from build123d import *

# Parameters (mm, degrees)
SALIENTE_EXTRUIR1_DEPTH = 5
CROQUIS2_R              = 2.5
SALIENTE_EXTRUIR2_DEPTH = 5
CROQUIS3_R              = 5
SALIENTE_EXTRUIR3_DEPTH = 10


with BuildPart() as part:
    # Croquis1 → Saliente-Extruir1 (new body)
    with BuildSketch(Plane.XY):
        with BuildLine():
            Line((-52.49750025, 5), (52.49750025, 5))
            Line((52.49750025, 5), (72.49750025, -10))
            Line((72.49750025, -10), (72.49750025, -25.5))
            Line((72.49750025, -25.5), (62.49750025, -25.5))
            Line((62.49750025, -25.5), (62.49750025, -12.5))
            Line((62.49750025, -12.5), (52.49750025, -5))
            Line((52.49750025, -5), (-52.49750025, -5))
            ThreePointArc((-52.49750025, -5), (-103.00249975, 0), (-52.49750025, 5))
        make_face()
    extrude(amount=SALIENTE_EXTRUIR1_DEPTH)

    # Croquis2 → Saliente-Extruir2 (add)
    with BuildSketch(Plane.XY.offset(5)):
        with Locations((-77.50249975, 12.5)):
            Circle(CROQUIS2_R)
    extrude(amount=SALIENTE_EXTRUIR2_DEPTH)

    # Croquis3 → Saliente-Extruir3 (add)
    with BuildSketch(Plane.XY.offset(5)):
        with Locations((-77.50249975, 0)):
            Circle(CROQUIS3_R)
    extrude(amount=SALIENTE_EXTRUIR3_DEPTH)


solid = part.part
Geometry check sheet. Reference: the model listing, model coordinates, mm. A direction names the side the tool comes from. Round coordinates to 2 decimals unless told otherwise and drop trailing zeros. Write each loop counter-clockwise with the first axis right and the second up, starting at its lowest first coordinate (ties: lowest second). Pieces come first, ordered by that corner, then holes. Notation, with made-up numbers: (-35, 76.5) -> (-28, 76.5) arc R25 cw to (-28, 93.5) -> close; hole circle Ø3 at (-20.5, -17.5). An arc over 180 degrees is marked (long way). One line per item, written item: value. Start each with the question number.
(1) Cross-section at D-D, the plane y = 18.5. Record the cut outline in (x, z).
(2) Access from +Z, -Z, +X, -X, +Y, -Y to the whole of each face (thin tool, end or side, straight path). Record for faces 4 (the flat face through (-78, 13, 10)), 5 (the cylindrical face through (-82.5, 0.2, 9.9)), 6 (the flat face through (57.568, -8.802, 2.465)).
(3) Cross-section at A-A, the plane z = 2.5. Record the cut outline in (x, y), and give its area (3 significant figures).
(4) Cross-section at C-C, the plane x = -40. Record the cut outline in (y, z), and give its area (3 significant figures).
(5) Scan lines: line 1 (Z direction, x = 14.5, y = -4.5); line 2 (Y direction, x = -22, z = 1.5); line 3 (X direction, y = -13.5, z = 2.5). Record each from-to range of solid material in increasing order. Write a range as [from, to].
(6) Draft check along Y on faces 1 (the cylindrical face through (-79.5, 11, 7.5)), 2 (the flat face through (-1, 5, 2)), 3 (the flat face through (62.498, -19, 2)). Enter one of: +Y half, -Y half, draft (parallel to the pull), parting line (faces both ways), or undercut.
(7) Cross-section at B-B, the plane y = 3. Record the cut outline in (x, z).
(8) Go/stop test with flat-tipped pins: pin 1 Ø2.5 at (x, z) = (-21.5, 3.5) entering from -Y; pin 2 Ø1.5 at (y, z) = (-20, 2.5) entering from -X; pin 3 Ø1.5 at (x, z) = (24.5, 3.5) entering from +Y. Record where each tip stops, or that it passes through.
Answer:
1. outline: (-95.05, 0) -> (-59.95, 0) -> (-59.95, 5) -> (-95.05, 5) -> close
2. face 4: +Z, +X, -X, +Y
2. face 5: +Z
2. face 6: +Z, -Z, -Y
3. outline: (-52.5, -5) -> (52.5, -5) -> (62.5, -12.5) -> (62.5, -25.5) -> (72.5, -25.5) -> (72.5, -10) -> (52.5, 5) -> (-52.5, 5) arc R25.5 ccw (long way) to start
3. area: 3,380 mm²
4. outline: (-5, 0) -> (5, 0) -> (5, 5) -> (-5, 5) -> close
4. area: 50.0 mm²
5. line 1: [0, 5]
5. line 2: [-5, 5]
5. line 3: [-99.14, -55.87], [62.5, 72.5]
6. face 1: undercut
6. face 2: +Y half
6. face 3: draft
7. outline: (-102.83, 0) -> (55.16, 0) -> (55.16, 5) -> (-73.5, 5) -> (-73.5, 15) -> (-81.5, 15) -> (-81.5, 5) -> (-102.83, 5) -> close
8. pin 1: y = -5
8. pin 2: x = -94.23
8. pin 3: y = 5
